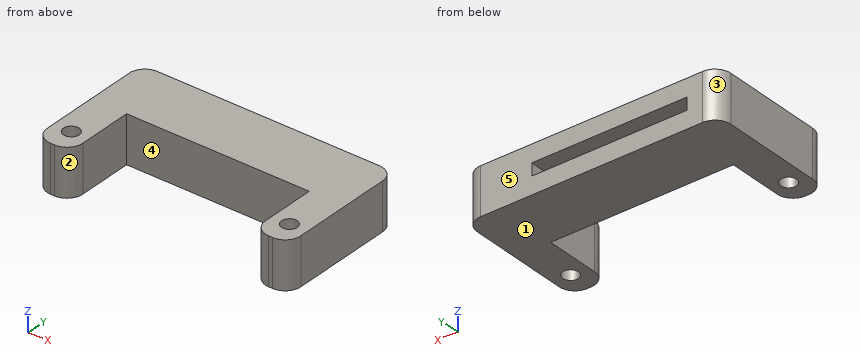
```python
from build123d import *

# Parameters (mm, degrees)
SKETCH2_W           = 32.2
SKETCH2_H           = 17.068
BOSS_EXTRUDE1_DEPTH = 3
SKETCH3_W           = 19.7
SKETCH3_H           = 1.55
CUT_EXTRUDE1_DEPTH  = 5
SKETCH4_W           = 23.2
SKETCH4_H           = 9
CUT_EXTRUDE2_DEPTH  = 20.18434664
SKETCH5_R           = 1
CUT_EXTRUDE3_DEPTH  = 20.18434664
FILLET1_R           = 2


with BuildPart() as part:
    # Sketch2 → Boss-Extrude1 (new, symmetric)
    with BuildSketch(Plane.XY):
        Rectangle(SKETCH2_W, SKETCH2_H)
    extrude(amount=BOSS_EXTRUDE1_DEPTH, both=True)

    # Sketch3 → Cut-Extrude1 (cut)
    with BuildSketch(Plane(origin=(0, 8.534, 0), x_dir=(1, 0, 0), z_dir=(0, 1, 0))):
        with Locations((-2.25, 0)):
            Rectangle(SKETCH3_W, SKETCH3_H)
    extrude(amount=-CUT_EXTRUDE1_DEPTH, mode=Mode.SUBTRACT)

    # Sketch4 → Cut-Extrude2 (cut, through all)
    with BuildSketch(Plane.XY.offset(3)):
        with Locations((0, -4.034)):
            Rectangle(SKETCH4_W, SKETCH4_H)
    extrude(amount=-CUT_EXTRUDE2_DEPTH, mode=Mode.SUBTRACT)

    # Sketch5 → Cut-Extrude3 (cut, through all)
    with BuildSketch(Plane.XY.offset(3)):
        with Locations((-13.85, -5.534)):
            Circle(SKETCH5_R)
        with Locations((13.85, -5.534)):
            Circle(SKETCH5_R)
    extrude(amount=-CUT_EXTRUDE3_DEPTH, mode=Mode.SUBTRACT)

    # Fillet1
    fillet1_edges = [part.edges().sort_by_distance(p)[0] for p in [
        (-11.6, -8.534, 0),
        (11.6, -8.534, 0),
        (16.1, -8.534, 0),
        (-16.1, -8.534, 0),
        (-16.1, 8.534, 0),
        (16.1, 8.534, 0),
    ]]
    fillet(fillet1_edges, radius=FILLET1_R)


solid = part.part
```
Check sheet for the modelled part. Datum: model origin and axes. Units: mm. Face numbers are marked on the shaded views. A direction names the side the tool comes from. Round coordinates to 2 decimals unless told otherwise and drop trailing zeros. Order: outer loops, then holes, each group sorted by start corner. A loop starts at its lowest first (then second) coordinate and runs counter-clockwise, first axis right, second up. Notation, with made-up numbers: (25.25, 48) - (76.25, 48) arc R16 cw to (76.25, 53) - close; hole circle Ø5 at (-23.5, -26). An arc over 180 degrees is marked (long way). Answer as CSV lines item,"result". Start each with the question number.
1) Draft check along X on the marked faces 1, 2 and 3. Enter one of: +X half, -X half, draft (parallel to the pull), parting line (faces both ways), or undercut.
2) Section check D-D (z = -2.2). Record the cut outline in (x, y).
3) Tool access check on the marked faces 4 and 5. Record the directions out of +Z, -Z, +X, -X, +Y, -Y that give a thin tool (end or side, any length) a straight path to the whole face; none if there is none.
4) Section check C-C (z = 0). Record the cut outline in (x, y).
5) Scan lines: probe 1 along X at (y, z) = (-5.5, 0.3); probe 2 along Y at (x, z) = (-13.85, -0.9); probe 3 along Z at (x, y) = (-12, 6.75) (3 decimals). Record each from-to range of solid material in increasing order.
6) Section check A-A (x = 7). Record the cut outline in (y, z) (3 decimals).
7) Depth check by flat-ended pin: pin 1 (3 mm diameter, centred on x = -2, z = -1.5, fed in from -Y); pin 2 (2 mm diameter, centred on x = 11, z = 0, fed in from -Y); pin 3 (1.2 mm diameter, centred on x = -5, z = 0, fed in from +Y). Enter the tip coordinate at first touch or a pass-through.
8) Section check B-B (y = -0.75). Record the cut outline in (x, z).
Determined:
1,face 1,"draft"
1,face 2,"undercut"
1,face 3,"-X half"
2,outline,"(-16.1, -6.53) arc R2 ccw to (-14.1, -8.53) - (-13.6, -8.53) arc R2 ccw to (-11.6, -6.53) - (-11.6, 0.47) - (11.6, 0.47) - (11.6, -6.53) arc R2 ccw to (13.6, -8.53) - (14.1, -8.53) arc R2 ccw to (16.1, -6.53) - (16.1, 6.53) arc R2 ccw to (14.1, 8.53) - (-14.1, 8.53) arc R2 ccw to (-16.1, 6.53) - close; hole circle Ø2 at (-13.85, -5.53); hole circle Ø2 at (13.85, -5.53)"
3,face 4,"+Z, -Z, -Y"
3,face 5,"+Z, -Z, +X, -X, +Y"
4,outline,"(-16.1, -6.53) arc R2 ccw to (-14.1, -8.53) - (-13.6, -8.53) arc R2 ccw to (-11.6, -6.53) - (-11.6, 0.47) - (11.6, 0.47) - (11.6, -6.53) arc R2 ccw to (13.6, -8.53) - (14.1, -8.53) arc R2 ccw to (16.1, -6.53) - (16.1, 6.53) arc R2 ccw to (14.1, 8.53) - (7.6, 8.53) - (7.6, 3.53) - (-12.1, 3.53) - (-12.1, 8.53) - (-14.1, 8.53) arc R2 ccw to (-16.1, 6.53) - close; hole circle Ø2 at (-13.85, -5.53); hole circle Ø2 at (13.85, -5.53)"
5,probe 1,"-16.1 to -14.85, -12.85 to -11.6, 11.6 to 12.85, 14.85 to 16.1"
5,probe 2,"-8.53 to -6.53, -4.53 to 8.53"
5,probe 3,"-3 to -0.775, 0.775 to 3"
6,outline,"(0.466, -3) - (8.534, -3) - (8.534, -0.775) - (3.534, -0.775) - (3.534, 0.775) - (8.534, 0.775) - (8.534, 3) - (0.466, 3) - close"
7,pin 1,"y = 0.47"
7,pin 2,"y = -7.73"
7,pin 3,"y = 3.53"
8,outline,"(-16.1, -3) - (-11.6, -3) - (-11.6, 3) - (-16.1, 3) - close; (11.6, -3) - (16.1, -3) - (16.1, 3) - (11.6, 3) - close"
